Could you check a few things on this model? Use its own coordinates, in mm. Face numbers are marked on the shaded views. A direction names the side the tool comes from. Give positions to 0.01 mm unless a question says otherwise; leave off trailing zeros. Order: outer loops, then holes, each group sorted by start corner. A loop starts at its lowest first (then second) coordinate and runs counter-clockwise, first axis right, second up.
(1) If we mould it in two halves opening along X, with no side actions, what happens to the marked faces 3, 4 and 5? For each: released by +X, released by -X, zero draft, split by the parting line, or undercut.
(2) Imagine slicing it at A-A, the plane z = 2.1. Write out the boundary of the cut face in (x, y), then the cut area to 3 significant figures.
(3) Imagine slicing it at B-B, the plane y = -15. Write out the boundary of the cut face in (x, z), then the cut area to 3 significant figures.
(4) Will this pin go through, and if not, where does the flat tip stop? pin 1 (1.5 mm diameter, centred on y = 2, z = 1, fed in from -X).
(5) Imagine slicing it at C-C, the plane x = 0. Write out the boundary of the cut face in (y, z).
(6) If I drill on probe 1 along Y at (x, z) = (0, 0.9); probe 2 along Y at (x, z) = (-6.25, 2.05); probe 3 along X at (y, z) = (1.5, 0.6), over which ranges is the centre line in solid material (lowest first)?
(7) Imagine slicing it at D-D, the plane y = 2. Write out the boundary of the cut face in (x, z).
(8) On a 3-axis mill with a long thin cutter (end or side, diameter ignored), from which of +Z, -Z, +X, -X, +Y, -Y can I reach the whole of each face in a straight line? I mean the marked faces 1 and 2. Say none if no direction works.
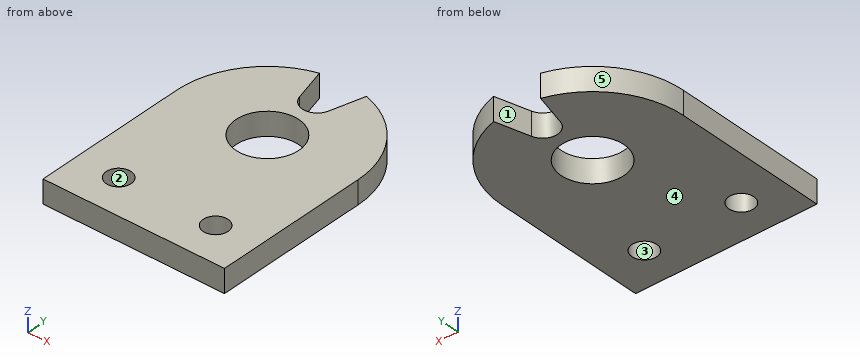
Autodesk Inventor part; units mm, degrees
ref_plane "YZ Plane" through (0, 0, 0) normal (1, 0, 0) x (0, 1, 0)
ref_plane "XZ Plane" through (0, 0, 0) normal (0, 1, 0) x (-1, 0, 0)
ref_plane "XY Plane" through (0, 0, 0) normal (0, 0, 1) x (1, 0, 0)
sketch "Sketch1" plane through (0, 0, 0) normal (0, 0, 1) x (1, 0, 0)
  arc A0 (-1.9, 11.5447) -> (-3.0282, 11.3013) centre (0, 0) ccw construction
  line L0 (0, 7.75) -> (0, 0) construction
  arc A1 (1.9, 11.5447) -> (-1.9, 11.5447) centre (0, 0) ccw construction
  circle A2 centre (0, 0) radius 4.05
  line L1 (11.7, 0) -> (11.7, -20)
  line L2 (11.7, -20) -> (-11.7, -20)
  line L3 (-11.7, -20) -> (-11.7, 0)
  arc A3 (11.7, 0) -> (3.0282, 11.3013) centre (0, 0) ccw
  arc A4 (-11.7, 0) -> (11.7, 0) centre (0, 0) ccw construction
  line L4 (3.0282, 11.3013) -> (1.872, 6.9864)
  line L5 (-1.872, 6.9864) -> (-3.0282, 11.3013)
  arc A5 (-1.872, 6.9864) -> (1.872, 6.9864) centre (0, 7.488) ccw
  arc A6 (3.0282, 11.3013) -> (1.9, 11.5447) centre (0, 0) ccw construction
  arc A7 (-3.0282, 11.3013) -> (-11.7, 0) centre (0, 0) ccw
  line L6 (-1.872, 6.9864) -> (0, 0) construction
  line L7 (0, 0) -> (1.872, 6.9864) construction
  line L8 (0, 5.55) -> (0, 4.05) construction
  dimension "d3" = 8.1
  dimension "d0" = 23.4
  dimension "d4" = 20
  dimension "d8" = 30
  dimension "d9" = 1.5
extrude "Extrusion1" add sketch "Sketch1" along normal blind 3
sketch "Sketch2" plane through (0, 0, 3) normal (0, 0, 1) x (1, 0, 0)
  circle A0 centre (-6.25, -15) radius 1.6
  circle A1 centre (6.25, -15) radius 1.6
  line L0 (-6.25, -15) -> (6.25, -15) construction
  line L1 (0, -15) -> (0, -20) construction
  line L2 (-11.7, -20) -> (11.7, -20) construction
  point P0 (0, 0)
  dimension "d10" = 3.2
  dimension "d11" = 5
  dimension "d12" = 12.5
extrude "Extrusion2" cut sketch "Sketch2" against normal through all
properties part number "Xgantry_CableChain_top_connector"
Answer block:
1. face 3: undercut
1. face 4: zero draft
1. face 5: released by -X
2. outline: (-11.7, -20) - (11.7, -20) - (11.7, 0) arc R11.7 ccw to (3.03, 11.3) - (1.87, 6.99) arc R1.94 cw to (-1.87, 6.99) - (-3.03, 11.3) arc R11.7 ccw to (-11.7, 0) - close; hole circle Ø3.2 at (-6.25, -15); hole circle Ø8.1 at (0, 0); hole circle Ø3.2 at (6.25, -15)
2. area: 589 mm2
3. outline: (-11.7, 0) - (-7.85, 0) - (-7.85, 3) - (-11.7, 3) - close; (-4.65, 0) - (4.65, 0) - (4.65, 3) - (-4.65, 3) - close; (7.85, 0) - (11.7, 0) - (11.7, 3) - (7.85, 3) - close
3. area: 51.0 mm2
4. pin 1: stops at x = -11.63
5. outline: (-20, 0) - (-4.05, 0) - (-4.05, 3) - (-20, 3) - close; (4.05, 0) - (5.55, 0) - (5.55, 3) - (4.05, 3) - close
6. probe 1: y = -20 to -4.05, 4.05 to 5.55
6. probe 2: y = -20 to -16.6, -13.4 to 9.89
6. probe 3: x = -11.6 to -3.76, 3.76 to 11.6
7. outline: (-11.53, 0) - (-3.52, 0) - (-3.52, 3) - (-11.53, 3) - close; (3.52, 0) - (11.53, 0) - (11.53, 3) - (3.52, 3) - close
8. face 1: +Z, -Z, +Y
8. face 2: +Z, -Z
